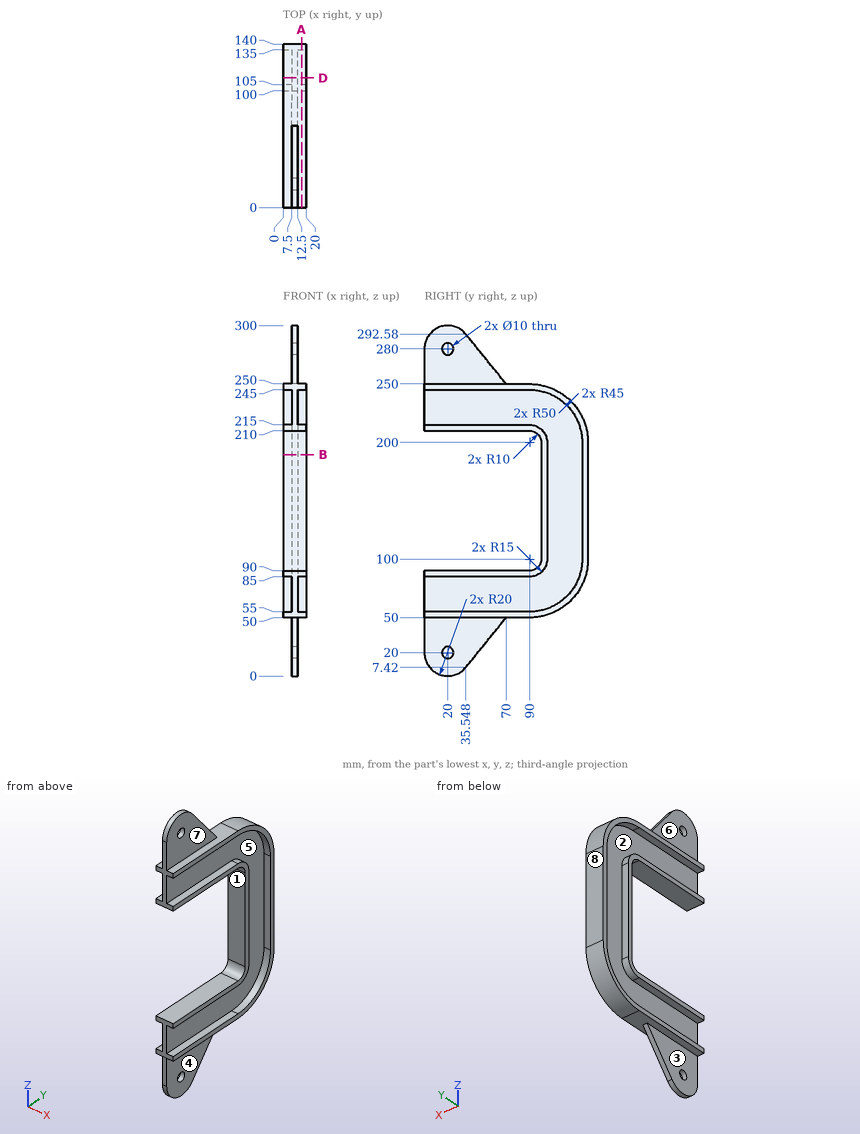
Drawing for the job (mm, zero at the part's lowest x, y, z). A direction names the side the tool comes from. Round coordinates to 2 decimals unless told otherwise and drop trailing zeros. Order: outer loops, then holes, each group sorted by start corner. A loop starts at its lowest first (then second) coordinate and runs counter-clockwise, first axis right, second up.
Item 1: Tool access for the marked faces 4, 5, 6, 7 and 8: list every direction of +Z, -Z, +X, -X, +Y, -Y with a clear straight run to the whole face (end or side of a thin tool).
Item 2: Saw through at A-A on x = 16. Write the cut outline in (y, z).
Item 3: Probe line 1 along Z through (x, y) = (7, 66.5); line 2 along Y through (x, z) = (2.75, 123); line 3 along Z through (x, y) = (11.5, 18.5). List the from-to ranges inside material, lowest first.
Item 4: Pin check, flat tips, straight feed: pin 1 (1.5 mm diameter, centred on x = 12, y = 85, fed in from -Z); pin 2 (10 mm diameter, centred on x = 12, y = 56, fed in from -Z); pin 3 (15 mm diameter, centred on y = 50.5, z = 23, fed in from -X). Stop position of each tip, or through.
Item 5: Saw through at D-D on y = 111. Write the cut outline in (x, z), then the cut area to 3 significant figures.
Item 6: Saw through at B-B on z = 189.5. Write the cut outline in (x, y), then the cut area to 3 significant figures.
Item 7: Mould opens along Y. For the marked faces 1, 2 and 3 say: pulls with the +Y half, pulls with the -Y half, needs draft (parallel to the pull), parting line crosses it, or undercut.
Reported:
1. face 4: -Z, +X, +Y, -Y
1. face 5: +X
1. face 6: +Z, -X, +Y, -Y
1. face 7: +Z, +X, +Y, -Y
1. face 8: +Z, -Z, +X, -X, +Y
2. outline: (0, 50) - (90, 50) arc R50 ccw to (140, 100) - (140, 200) arc R50 ccw to (90, 250) - (0, 250) - (0, 245) - (90, 245) arc R45 cw to (135, 200) - (135, 100) arc R45 cw to (90, 55) - (0, 55) - close; (0, 85) - (90, 85) arc R15 ccw to (105, 100) - (105, 200) arc R15 ccw to (90, 215) - (0, 215) - (0, 210) - (90, 210) arc R10 cw to (100, 200) - (100, 100) arc R10 cw to (90, 90) - (0, 90) - close
3. line 1: z = 50 to 55, 85 to 90, 210 to 215, 245 to 250
3. line 2: y = 100 to 105, 135 to 140
3. line 3: z = 0.06 to 15.23, 24.77 to 90, 210 to 275.23, 284.77 to 299.94
4. pin 1: stops at z = 50
4. pin 2: stops at z = 26.52
4. pin 3: stops at x = 7.5
5. outline: (0, 54.62) - (20, 54.62) - (20, 60.2) - (12.5, 60.2) - (12.5, 239.8) - (20, 239.8) - (20, 245.38) - (0, 245.38) - (0, 239.8) - (7.5, 239.8) - (7.5, 60.2) - (0, 60.2) - close
5. area: 1,120 mm2
6. outline: (0, 100) - (20, 100) - (20, 105) - (12.5, 105) - (12.5, 135) - (20, 135) - (20, 140) - (0, 140) - (0, 135) - (7.5, 135) - (7.5, 105) - (0, 105) - close
6. area: 350 mm2
7. face 1: pulls with the -Y half
7. face 2: undercut
7. face 3: needs draft
